Part model, mm, in its own coordinate system. A direction names the side the tool comes from. Give positions to 0.01 mm unless a question says otherwise; leave off trailing zeros. Loops run counter-clockwise (first coordinate to the right, second up) from the corner with the lowest first, then second, coordinate; pieces in that order, holes last. Notation, with made-up numbers: (-38.5, 80) -> (0.5, 80) arc R29 ccw to (0.5, 111) -> close; hole circle Ø7 at (15, 2.25). An arc over 180 degrees is marked (long way). Write item = value, one per line.
from build123d import *

# Parameters (mm, degrees)
SKETCH_1_R          = 7
EXTRUDE_1_DEPTH     = 10
SKETCH_9_W          = 5.615402883
SKETCH_9_H          = 4.534999238
EXTRUDE_6_DEPTH     = 1
SKETCH_11_W         = 1.257653538
SKETCH_11_H         = 9
EXTRUDE_7_DEPTH     = 4.5
EXTRUDE_8_DEPTH     = 6
FILLET_8_R          = 1
FILLET_9_R          = 1
SKETCH_14_W         = 3.266646727
SKETCH_14_H         = 7
CUT_EXTRUDE_1_DEPTH = 10
CUT_EXTRUDE_START   = -2
CUT_EXTRUDE_2_DEPTH = 2
CUT_EXTRUDE_3_DEPTH = 2
SKETCH_17_W         = 6
SKETCH_17_H         = 6.96519698
CUT_EXTRUDE_5_DEPTH = 2


with BuildPart() as part:
    # Sketch 1 → Extrude 1 (new body)
    with BuildSketch(Plane(origin=(0.382706605, 0, 0), x_dir=(1, 0, 0), z_dir=(0, 0, 1))):
        with Locations((-75.594417438, 2.55)):
            Circle(SKETCH_1_R)
    extrude(amount=EXTRUDE_1_DEPTH)

    # Sketch 9 → Extrude 6 (add)
    with BuildSketch(Plane(origin=(8.106794936, 0, 9), x_dir=(1, 0, 0), z_dir=(0, 0, 1))):
        with Locations((-74.892231202, 2.267499619)):
            Rectangle(SKETCH_9_W, SKETCH_9_H)
    extrude(amount=EXTRUDE_6_DEPTH)



with BuildPart() as body_2:
    # Sketch 11 → Extrude 7 (new body)
    with BuildSketch(Plane(origin=(11.553490323, 4.534999238, 0.48426017), x_dir=(1, 0, 0), z_dir=(0, 1, 0))):
        with Locations((-76.184774061, -4.5)):
            Rectangle(SKETCH_11_W, SKETCH_11_H)
    extrude(amount=-EXTRUDE_7_DEPTH)


with BuildPart() as part_1:
    add(part.part)

    add(body_2.part)  # Extrude 8 merges body 2
    # Sketch 12 → Extrude 8 (add)
    with BuildSketch(Plane.ZY.offset(65.260110507)):
        Polygon((0.48426017, 4.534999238), (0.48426017, 0), (1.483647509, 0.034999238), (1.483647509, 4.534999238), align=None)
    extrude(amount=EXTRUDE_8_DEPTH)

    # Fillet 8
    fillet_8_edges = [part_1.edges().sort_by_distance(p)[0] for p in [
        (-64.002456969, 2.284999238, 0.48426017),
    ]]
    fillet(fillet_8_edges, radius=FILLET_8_R)

    # Fillet 9
    fillet_9_edges = [part_1.edges().sort_by_distance(p)[0] for p in [
        (-63.977734824, 2.267499619, 10),
    ]]
    fillet(fillet_9_edges, radius=FILLET_9_R - 0.0001)  # a hair under: the kernel refuses the full size

    # Sketch 14 → Cut-Extrude 1 (cut)
    with BuildSketch(Plane.XY.offset(10)):
        with Locations((-77.998959421, 2.53259849)):
            Rectangle(SKETCH_14_W, SKETCH_14_H)
    extrude(amount=-CUT_EXTRUDE_1_DEPTH, mode=Mode.SUBTRACT)

    # Sketch 15 → Cut-Extrude 2 (cut)
    with BuildSketch(Plane.XY.offset(10).offset(CUT_EXTRUDE_START)):
        with BuildLine():
            Line((-79.632282784, 6.03259849), (-81.28390218, 6.03259849))
            ThreePointArc((-81.28390218, 6.03259849), (-82.211710833, 2.55), (-81.28390218, -0.93259849))
            Line((-81.28390218, -0.93259849), (-79.632282784, -0.96740151))
            Line((-79.632282784, -0.96740151), (-79.632282784, 6.03259849))
        make_face()
    extrude(amount=CUT_EXTRUDE_2_DEPTH, mode=Mode.SUBTRACT)

    # Sketch 16 → Cut-Extrude 3 (cut)
    with BuildSketch(Plane(origin=(0, 0, 0), x_dir=(-1, 0, 0), z_dir=(0, 0, -1))):
        with BuildLine():
            Line((79.632282784, 6.03259849), (81.28390218, 6.03259849))
            ThreePointArc((81.28390218, 6.03259849), (82.211710833, 2.55), (81.28390218, -0.93259849))
            Line((81.28390218, -0.93259849), (79.632282784, -0.96740151))
            Line((79.632282784, -0.96740151), (79.632282784, 6.03259849))
        make_face()
    extrude(amount=-CUT_EXTRUDE_3_DEPTH, mode=Mode.SUBTRACT)

    # Sketch 17 → Cut-Extrude 5 (cut)
    with BuildSketch(Plane.ZY.offset(83.365636057)):
        with Locations((5, 2.55)):
            Rectangle(SKETCH_17_W, SKETCH_17_H)
    extrude(amount=-CUT_EXTRUDE_5_DEPTH, mode=Mode.SUBTRACT)


solid = part_1.part
1) Drill centre lines: line 1 along X through (y, z) = (2.5, 3); line 2 along X through (y, z) = (0.5, 7.5); line 3 along X through (y, z) = (5.5, 7.5). Where is each one in solid material? Low to high. Write a range as [from, to].
Resolved:
line_1 = [-81.37, -79.63], [-76.37, -68.21], [-65.26, -64]
line_2 = [-81.37, -79.63], [-76.37, -68.52], [-65.26, -64]
line_3 = [-81.37, -79.63], [-76.37, -68.86]
2) Slice it at D-D, the plane y = 5. List the corners of the cut face in (x, z), and give its area (3 significant figures).
Resolved:
outline = (-81.37, 2) -> (-79.63, 2) -> (-79.63, 8) -> (-81.37, 8) -> close; (-76.37, 0) -> (-68.65, 0) -> (-68.65, 10) -> (-76.37, 10) -> close
area = 87.5 mm²
3) Drop flat-ended pins along their axis: P1, Ø1.3, axis at y = 2.5, z = 4, coming from the +X side; P2, Ø0.8, axis at x = -66, z = 9.5, coming from the -Y side; P3, Ø1.5, axis at y = 7.5, z = 8.5, coming from the -X side. Give the stop position or say it passes through.
Resolved:
P1 = -64
P2 = 0
P3 = -80.81
4) Pull direction Z, two halves, no side cores. Call faces 1 (the face through (-65, 0.035, 5)), 2 (the face through (-67, 2, 1.484)), 3 (the face through (-67, 2, 0.484)): pulls with the +Z half, pulls with the -Z half, needs draft (parallel to the pull), parting line crosses it, or undercut.
Resolved:
face_1 = needs draft
face_2 = undercut
face_3 = pulls with the -Z half
5) Slice it at C-C, the plane x = -67.5. List the corners of the cut face in (y, z) (3 decimals), and give its area (3 significant figures).
Resolved:
outline = (0, 0.484) -> (4.535, 0.484) -> (4.535, 1.484) -> (0.035, 1.484) -> close; (0, 9) -> (4.535, 9) -> (4.535, 10) -> (0, 10) -> close
area = 9.05 mm²
6) Which spindle directions (+Z, -Z, +X, -X, +Y, -Y) get a long thin tool onto all of the face, cutting with end or side? Do faces 4 (the face through (-65, 4.535, 5)), 5 (the face through (-66.4, 0, 9.5)), 6 (the face through (-79.632, 2, 5)). Say none if no direction does.
Resolved:
face_4 = +Z, -Z, +X, +Y
face_5 = +Z, -Z, +X, -Y
face_6 = +Z, -Z
7) Slice it at B-B, the plane z = 7.75. List the corners of the cut face in (x, y) (3 decimals).
Resolved:
outline = (-81.366, -0.786) arc R7 ccw (long way) to (-81.366, 5.886) -> close; (-65.26, 0.035) -> (-64.002, 0.035) -> (-64.002, 4.535) -> (-65.26, 4.535) -> close; hole (-79.632, -0.967) -> (-76.366, -0.967) -> (-76.366, 6.033) -> (-79.632, 6.033) -> close
8) Slice it at A-A, the plane y = 2.55. Count the separate pieces of the cut face and the enclosed holes in it, and give its area (3 significant figures).
Resolved:
separate_pieces = 2
enclosed_holes = 1
area = 109 mm²
